Input: part model. Units: mm. Frame: model coordinates. Face numbers are marked on the shaded views. A direction names the side the tool comes from. Round coordinates to 2 decimals unless told otherwise and drop trailing zeros. Order: outer loops, then holes, each group sorted by start corner. A loop starts at its lowest first (then second) coordinate and runs counter-clockwise, first axis right, second up. Notation, with made-up numbers: (40.5, -37.75) - (68.5, -37.75) arc R16 ccw to (68.5, -26.75) - close; hole circle Ø9 at (17, 56). An arc over 180 degrees is marked (long way). One line per item, written item: value. Start each with the question number.
from build123d import *

# Parameters (mm, degrees)
F2_SIZE2 = 1.154701
F2_SIZE  = 2
F3_R     = 2.5
F4_DEPTH = 6
F5_SIZE2 = 1.154701
F5_SIZE  = 2
F6_SIZE  = 1


with BuildPart() as f1:
    # F0 (on Front) → F1 (revolve)
    with BuildSketch(Plane.XZ):
        Polygon((-148.261028, 17.5), (-141.261028, 17.5), (-141.261028, 39.425), (-145.661028, 39.425), (-145.661028, 38), (-149.261028, 38), (-149.261028, 31), (-171.761028, 31), (-171.761028, 38), (-175.361028, 38), (-175.361028, 39.425), (-186.261028, 39.425), (-186.261028, 16), (-154.261028, 16), (-154.261028, 17.5), (-150.961028, 17.5), (-150.961028, 19.95), (-148.261028, 19.95), align=None)
    revolve(axis=Axis((28.175471, 0, 0), (1, 0, 0)))

    # F2
    f2_edges = [f1.edges().sort_by_distance(p)[0] for p in [
        (-186.261028, 0, -39.425),
    ]]
    chamfer(f2_edges, length=F2_SIZE, length2=F2_SIZE2)

    # F3 (on face) → F4 (cut)
    with BuildSketch(Plane(origin=(-186.261028, 0, 0), x_dir=(0, -1, 0), z_dir=(-1, 0, 0))):
        with Locations((0, 27)):
            Circle(F3_R)
        with Locations((0, -27)):
            Circle(F3_R)
    extrude(amount=-F4_DEPTH, mode=Mode.SUBTRACT)

    # F5
    f5_edges = [f1.edges().sort_by_distance(p)[0] for p in [
        (-141.261028, 0, -39.425),
    ]]
    chamfer(f5_edges, length=F5_SIZE, length2=F5_SIZE2)

    # F6
    f6_edges = [f1.edges().sort_by_distance(p)[0] for p in [
        (-186.261028, 0, -16),
        (-141.261028, 0, -17.5),
    ]]
    chamfer(f6_edges, length=F6_SIZE)


solid = f1.part
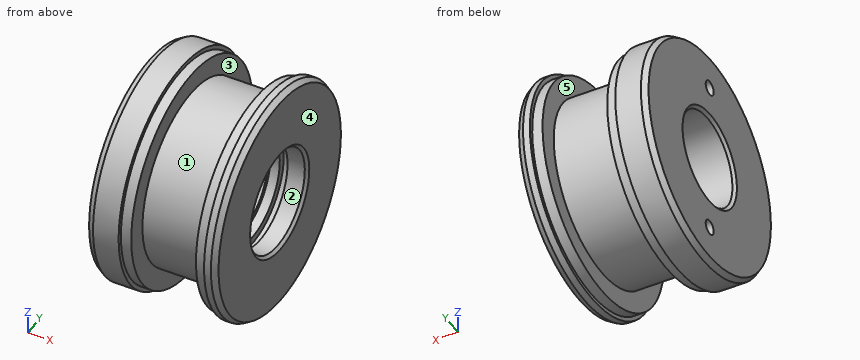
Item 1: Section query A-A on x = -162.5. Return loops of the section in (y, z).
Item 2: Line query: L1, parallel to Z at x = -181.5, y = 0 (3 decimals); L2, parallel to Y at x = -152, z = 0. Output: solid intervals per line, ascending.
Item 3: Pull-direction query (Z, two-part tool) for the marked faces 1, 2 and 3; classes: released by +Z, released by -Z, zero draft, split by the parting line, or undercut.
Item 4: First-contact query: pin 1 Ø1.5 at (y, z) = (0.5, 26.5) entering from -X; pin 2 Ø1.5 at (x, y) = (-162, 5.5) entering from -Z; pin 3 Ø4 at (x, z) = (-155, 28) entering from +Y. Flat tips, straight axial feed; report the tip coordinate or a pass-through.
Item 5: Reachability of the marked faces 4 and 5 from +Z, -Z, +X, -X, +Y, -Y: full face, straight path, thin tool, end or side. Return the list, or none.
Item 6: Section query B-B on x = -179. Return loops of the section in (y, z) (3 decimals).
Geometry results:
1. outline: circle Ø62 at (0, 0); hole circle Ø32 at (0, 0)
2. L1: z = -39.425 to -29.5, -24.5 to -16, 16 to 24.5, 29.5 to 39.425
2. L2: y = -31 to -17.5, 17.5 to 31
3. face 1: split by the parting line
3. face 2: undercut
3. face 3: zero draft
4. pin 1: stops at x = -180.26
4. pin 2: stops at z = -30.63
4. pin 3: stops at y = 16.88
5. face 4: +Z, -Z, +X, +Y, -Y
5. face 5: none
6. outline: circle Ø78.85 at (0, 0); hole circle Ø32 at (0, 0)
